Here's the drawing with two shaded views (mm, measured from the low corner). I have some questions. A direction names the side the tool comes from. Give positions to 0.01 mm unless a question says otherwise; leave off trailing zeros. Order: outer loops, then holes, each group sorted by start corner. A loop starts at its lowest first (then second) coordinate and runs counter-clockwise, first axis right, second up. Notation, with made-up numbers: M 88,-26.5 L 145,-26.5 A23 cw 145,5.5 Z; hole C -35.5,-35.75 d8. An arc over 180 degrees is marked long. One line per question, with ' | ' between items. Start each with the question number.
1) Please list where these lines run through material, in increasing order: line 1 along Z through (x, y) = (38.1, 3.25); line 2 along Y through (x, z) = (44.5, 4.75); line 3 along Z through (x, y) = (12, 19.5). Write a range as [from, to].
2) For the marked faces 4 and 5, which set-ups out of +Z, -Z, +X, -X, +Y, -Y let a thin tool reach every point of the face, with its end or its side?
3) I'm going to push flat-ended pins straight in: pin 1 Ø7.5 at (x, z) = (38.1, 15.875) entering from +Y; pin 2 Ø4 at (x, y) = (29, 22.5) entering from +Z. Where does each tip first touch, or does it pass through?
4) If we section it at C-C, the plane z = 4.5: State how many separate pieces and enclosed holes the cut face has, plus the area to 3 significant figures.
5) If we section it at A-A, the plane x = 38.1: Please give me the cut outline in (y, z), plus the area to 3 significant figures.
6) Thinking about a two-plate mould opening in Z: for the marked faces 1, 2 and 3, which applies, +Z half, -Z half, draft (parallel to the pull), parting line (faces both ways), or undercut?
7) If we section it at B-B, the plane y = 15: Please give me the cut outline in (x, z).
8) If we section it at D-D, the plane x = 44.45: Please give me the cut outline in (y, z).
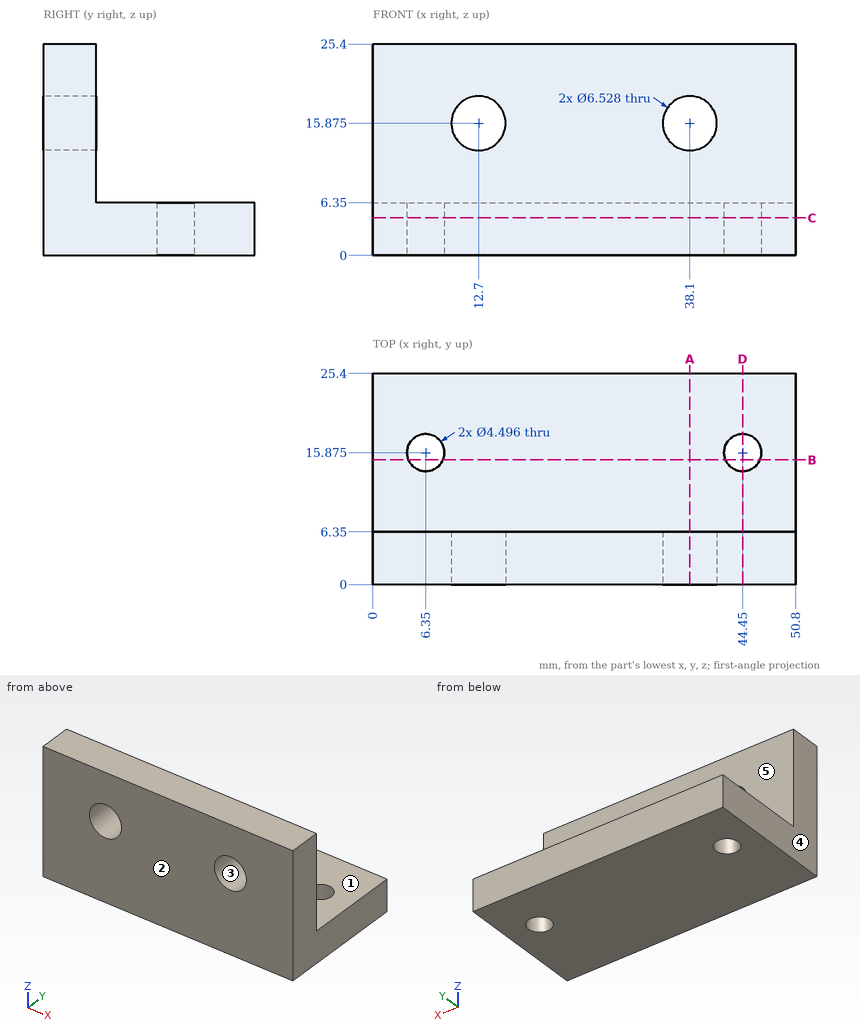
Results found:
1) line 1: z = [0, 12.61], [19.14, 25.4] | line 2: y = [0, 13.63], [18.12, 25.4] | line 3: z = [0, 6.35]
2) face 4: +Z, -Z, -X, +Y, -Y | face 5: +Z, +X, -X, +Y
3) pin 1: stops at y = 6.35 | pin 2: stops at z = 6.35
4) separate pieces: 1 | enclosed holes: 2 | area: 1,260 mm²
5) outline: M 0,0 L 25.4,0 L 25.4,6.35 L 6.35,6.35 L 6.35,12.61 L 0,12.61 Z; M 0,19.14 L 6.35,19.14 L 6.35,25.4 L 0,25.4 Z | area: 241 mm²
6) face 1: +Z half | face 2: draft | face 3: undercut
7) outline: M 0,0 L 4.28,0 L 4.28,6.35 L 0,6.35 Z; M 8.42,0 L 42.38,0 L 42.38,6.35 L 8.42,6.35 Z; M 46.52,0 L 50.8,0 L 50.8,6.35 L 46.52,6.35 Z
8) outline: M 0,0 L 13.63,0 L 13.63,6.35 L 6.35,6.35 L 6.35,25.4 L 0,25.4 Z; M 18.12,0 L 25.4,0 L 25.4,6.35 L 18.12,6.35 Z
